Part model, mm, in its own coordinate system. A direction names the side the tool comes from. Coordinates: 2 decimals unless noted, no trailing zeros. Loops run counter-clockwise (first coordinate to the right, second up) from the corner with the lowest first, then second, coordinate; pieces in that order, holes last. Notation, with made-up numbers: (2, -37.75) - (36, -37.75) arc R21 cw to (36, -12.75) - close; hole circle Ø3 at (-35.75, -34). An arc over 180 degrees is marked (long way). Use a Markdown table: item, result. Add a question column.
1) Probe probe 1 along X at (y, z) = (-1, 0); probe 2 along Y at (x, z) = (3.5, -0.25); probe 3 along X at (y, z) = (-4.5, 0.75). List the from-to ranges inside material, lowest first. Write a range as [from, to].
2) Band-saw the part on A-A (z = 0). Give the cut face in (x, y).
3) Band-saw the part on B-B (y = 0). Give the cut face in (x, z), plus the area to 3 significant figures.
4) Band-saw the part on C-C (x = 8). Give the cut face in (y, z), plus the area to 3 significant figures.
5) Band-saw the part on D-D (y = -2.75). Give the cut face in (x, z).
6) Tool access for faces 1 (the face through (-2.639, -3.135, -2.404)), 2 (the face through (18.896, 3.695, -1.532)), 3 (the face through (-15.499, 0, 0)), 4 (the face through (-12.956, -3.746, 0.165)): list every direction of +Z, -Z, +X, -X, +Y, -Y with a clear straight run to the whole face (end or side of a thin tool).
7) Drop flat-ended pins along their axis: P1, Ø6, axis at x = 0, z = -2.5, coming from the +Y side; P2, Ø6, axis at x = 2, z = -2.5, coming from the -Y side; P3, Ø5, axis at x = 15, z = 2.5, coming from the +Y side. Give the stop position or say it passes through.
8) Pull direction X, two halves, no side cores. Call faces 5 (the face through (26.501, 0, 0)), 6 (the face through (24.454, 0.056, -0.3)), 7 (the face through (-14.464, -3.135, -2.404)): +X half, -X half, draft (parallel to the pull), parting line (faces both ways), or undercut.
from build123d import *

# Parameters (mm, degrees)
SKETCH_2_R          = 1
CUT_EXTRUDE_1_DEPTH = 5


with BuildPart() as part:
    # 草图1 → 旋转1 (revolve)
    with BuildSketch(Plane.XY):
        Polygon((-15.499429975, 0), (26.500570025, 0), (26.500570025, 4), (11.500570025, 4), (11.500570025, 5), (7.500570025, 5), (7.500570025, 3.95), (-12.499429975, 3.95), (-12.499429975, 3.75), (-13.399429975, 3.75), (-13.399429975, 3.95), (-15.499429975, 3.95), align=None)
    revolve(axis=Axis((-15.499429975, 0, 0), (1, 0, 0)))

    # 草图2 → 切除-拉伸1 (cut, symmetric)
    with BuildSketch(Plane(origin=(0, 0, 0), x_dir=(1, 0, 0), z_dir=(0, 1, 0))):
        with Locations((23.500570025, 0)):
            Circle(SKETCH_2_R)
    extrude(amount=CUT_EXTRUDE_1_DEPTH, both=True, mode=Mode.SUBTRACT)


solid = part.part
Answer block:
| question | item | result |
|---|---|---|
| 1 | probe 1 | [-15.5, 22.5], [24.5, 26.5] |
| 1 | probe 2 | [-3.94, 3.94] |
| 1 | probe 3 | [7.5, 11.5] |
| 2 | outline | (-15.5, -3.95) - (-13.4, -3.95) - (-13.4, -3.75) - (-12.5, -3.75) - (-12.5, -3.95) - (7.5, -3.95) - (7.5, -5) - (11.5, -5) - (11.5, -4) - (22.5, -4) - (22.5, 4) - (11.5, 4) - (11.5, 5) - (7.5, 5) - (7.5, 3.95) - (-12.5, 3.95) - (-12.5, 3.75) - (-13.4, 3.75) - (-13.4, 3.95) - (-15.5, 3.95) - close; (24.5, -4) - (26.5, -4) - (26.5, 4) - (24.5, 4) - close |
| 3 | outline | (-15.5, -3.95) - (-13.4, -3.95) - (-13.4, -3.75) - (-12.5, -3.75) - (-12.5, -3.95) - (7.5, -3.95) - (7.5, -5) - (11.5, -5) - (11.5, -4) - (26.5, -4) - (26.5, 4) - (11.5, 4) - (11.5, 5) - (7.5, 5) - (7.5, 3.95) - (-12.5, 3.95) - (-12.5, 3.75) - (-13.4, 3.75) - (-13.4, 3.95) - (-15.5, 3.95) - close; hole circle Ø2 at (23.5, 0) |
| 3 | area | 338 mm2 |
| 4 | outline | circle Ø10 at (0, 0) |
| 4 | area | 78.5 mm2 |
| 5 | outline | (-15.5, -2.84) - (-13.4, -2.84) - (-13.4, -2.55) - (-12.5, -2.55) - (-12.5, -2.84) - (7.5, -2.84) - (7.5, -4.18) - (11.5, -4.18) - (11.5, -2.9) - (26.5, -2.9) - (26.5, 2.9) - (11.5, 2.9) - (11.5, 4.18) - (7.5, 4.18) - (7.5, 2.84) - (-12.5, 2.84) - (-12.5, 2.55) - (-13.4, 2.55) - (-13.4, 2.84) - (-15.5, 2.84) - close; hole circle Ø2 at (23.5, 0) |
| 6 | face 1 | -X |
| 6 | face 2 | +X |
| 6 | face 3 | +Z, -Z, -X, +Y, -Y |
| 6 | face 4 | none |
| 7 | P1 | y = 3.95 |
| 7 | P2 | y = -3.95 |
| 7 | P3 | y = 4 |
| 8 | face 5 | +X half |
| 8 | face 6 | undercut |
| 8 | face 7 | draft |
